For this review, take the finished solid that the model builds, in its own axes (mm). Give positions to 0.01 mm unless a question says otherwise; leave off trailing zeros. Loops run counter-clockwise (first coordinate to the right, second up) from the corner with the lowest first, then second, coordinate; pieces in that order, holes last. Notation, with made-up numbers: (-37, -17.5) - (-27, -17.5) arc R15 ccw to (-27, -1.5) - close; hole circle Ø8 at (-9.5, -2.75). An arc over 180 degrees is marked (long way). Use CSV: the item, a comma, the result in double quotes. Start each with the question number.
1. Take a section at A-A on y = 26. Give the boundary of the cut face in (x, z), plus the area to 3 significant figures.
2. Wall thickness on line 1 (X direction, y = 34.5, z = 21.25); line 2 (Z direction, x = 0.25, y = 18.5); line 3 (Z direction, x = 1.25, y = 21.5): over which ranges is each line inside the solid? List them lowest first.
3. For pin 1 (5 mm diameter, centred on x = -2.5, y = 30, fed in from +Z); pin 2 (2 mm diameter, centred on x = -4.5, y = 37.5, fed in from +Z); pin 3 (2 mm diameter, centred on y = 21, z = 24, fed in from +X); pin 4 (4 mm diameter, centred on y = 38.5, z = 18, fed in from -X), all flat-tipped, find the tip position at first contact; note any pin that passes through.
Autodesk Fusion 360 part; units mm, degrees
sketch "PinWay" plane through (0, 65, 0) normal (0, 1, 0) x (1, 0, 0)
  line L0 (0, 0) -> (0, -30) construction
  line L1 (0, -30) -> (4.125, -30)
  line L2 (4.125, -30) -> (4.125, -25.8571)
  line L3 (-4.125, -30) -> (-4.125, -25.8571)
  line L4 (0, -30) -> (-4.125, -30)
  arc A0 (4.125, -25.8571) -> (-4.125, -25.8571) centre (0, -21.5) ccw
  circle A1 centre (0, -21.5) radius 5.5
  circle A2 centre (0, -21.5) radius 3
  dimension "d1" = 0
  dimension "d2" = 0
  dimension "d3" = 0
  dimension "d4" = 0
  dimension "d5" = 0
  dimension "d6" = 0
extrude "Extrude1" add sketch "PinWay" against normal blind 49 contours A1 | A2
extrude "Extrude2" cut 1 faces at (0.5081, 65, 24.6232) along direction (0, -1, 0) blind 24
chamfer "Chamfer1" distance 0.8 angle 45 2 edges at (-5.1278, 41, 19.5111) (-5.1278, 16, 19.5111)
equation "d156 = TopPinBlank"
equation "d158 = TopPinBlank + TopPinLength"
equation "TopPinLength = 25 mm"
equation "TopPinBlank = -49 mm"
equation "d1 = PinWayDiameter"
equation "d2 = PinWayDepth"
equation "d3 = BodyThickness"
equation "d4 = PinWayOpening / 2"
equation "d5 = Pin"
equation "d6 = SpoolPinCenter"
Check result:
1,outline,"circle Ø11 at (0, 21.5)"
1,area,"95.0 mm²"
2,line 1,"x = -5.49 to 5.49"
2,line 2,"z = 16.01 to 26.99"
2,line 3,"z = 16.14 to 26.86"
3,pin 1,"stops at z = 27"
3,pin 2,"stops at z = 25.74"
3,pin 3,"stops at x = 5.29"
3,pin 4,"stops at x = -5.29"
